Here's how the part is built. I have some questions about the finished solid (model axes, mm). A direction names the side the tool comes from. Coordinates: 2 decimals unless noted, no trailing zeros. Order: outer loops, then holes, each group sorted by start corner. A loop starts at its lowest first (then second) coordinate and runs counter-clockwise, first axis right, second up. Notation, with made-up numbers: (26.5, 80.5) - (56.5, 80.5) arc R18 cw to (56.5, 99.5) - close; hole circle Ø3 at (42, 66). An arc over 180 degrees is marked (long way). Answer in a Markdown table with one row per item. Add a question column.
Item 1: On a 3-axis mill with a long thin cutter (end or side, diameter ignored), from which of +Z, -Z, +X, -X, +Y, -Y can I reach the whole of each face in a straight line? I mean faces 1 (the flat face through (-2.4, -1, 0)), 2 (the flat face through (2.4, -1, 0)), 3 (the flat face through (-1, -2, 1)). Say none if no direction works.
Item 2: If I drill on line 1 along Z through (x, y) = (0, 0.5); line 2 along X through (y, z) = (-0.55, 0); line 3 along Y through (x, z) = (-5.5, 0.6), over which ranges is the centre line in solid material (lowest first)? Write a range as from..to.
Item 3: Thinking about a two-plate mould opening in Z: for faces 4 (the flat face through (0, 1, -3)), 5 (the cylindrical face through (-0.27, 0.28, 1.22)), 6 (the flat face through (0, 1, 3)), 7 (the flat face through (-6, 1, 0)), which applies, +Z half, -Z half, draft (parallel to the pull), parting line (faces both ways), or undercut?
Item 4: I want a section at D-D (z = -2.15). Please give me the cut outline in (x, y).
Item 5: I want a section at A-A (x = 0). Please give me the cut outline in (y, z), plus the area to 4 significant figures.
Item 6: Will these pins go through, and if not, where does the flat tip stop? pin 1 Ø1 at (y, z) = (-1, 1) entering from +X; pin 2 Ø1 at (x, z) = (4, -1) entering from -Y.
Item 7: I want a section at B-B (y = -1.7). Please give me the cut outline in (x, z), plus the area to 3 significant figures.
Item 8: I want a section at C-C (z = 0). Please give me the cut outline in (x, y), plus the area to 4 significant figures.
```python
from build123d import *

# Parameters (mm, degrees)
BOSS_EXTRU_1_DEPTH      = 3
ESQUISSE2_R             = 1.25
ENL_V_MAT_EXTRU_1_DEPTH = 5.5
CONG_1_R                = 0.5


with BuildPart() as part:
    # Esquisse1 → Boss.-Extru.1 (new body, symmetric)
    with BuildSketch(Plane.XY):
        Polygon((-6, 0), (-2.4, 0), (-2.4, -2), (2.4, -2), (2.4, 0), (6, 0), (6, 2.5), (-6, 2.5), align=None)
    extrude(amount=BOSS_EXTRU_1_DEPTH, both=True)

    # Esquisse2 → Enlèv. mat.-Extru.1 (cut, through all)
    with BuildSketch(Plane(origin=(0, 2.5, 0), x_dir=(1, 0, 0), z_dir=(0, 1, 0))):
        Circle(ESQUISSE2_R)
    extrude(amount=-ENL_V_MAT_EXTRU_1_DEPTH, mode=Mode.SUBTRACT)

    # Congé1
    cong_1_edges = [part.edges().sort_by_distance(p)[0] for p in [
        (-6, 1.25, -3),
        (6, 1.25, -3),
        (-6, 1.25, 3),
        (-2.4, -1, 3),
        (2.4, -1, 3),
        (6, 1.25, 3),
        (2.4, -1, -3),
        (-2.4, -1, -3),
    ]]
    fillet(cong_1_edges, radius=CONG_1_R)


solid = part.part
```
Values follow:
| question | item | result |
|---|---|---|
| 1 | face 1 | +Z, -Z, -X, -Y |
| 1 | face 2 | +Z, -Z, +X, -Y |
| 1 | face 3 | +Z, -Z, +X, -X, -Y |
| 2 | line 1 | z = -3..-1.25, 1.25..3 |
| 2 | line 2 | x = -2.4..-1.25, 1.25..2.4 |
| 2 | line 3 | y = 0..2.5 |
| 3 | face 4 | -Z half |
| 3 | face 5 | undercut |
| 3 | face 6 | +Z half |
| 3 | face 7 | draft |
| 4 | outline | (-6, 0) - (-2.4, 0) - (-2.4, -2) - (2.4, -2) - (2.4, 0) - (6, 0) - (6, 2.5) - (-6, 2.5) - close |
| 5 | outline | (-2, -3) - (2.5, -3) - (2.5, -1.25) - (-2, -1.25) - close; (-2, 1.25) - (2.5, 1.25) - (2.5, 3) - (-2, 3) - close |
| 5 | area | 15.75 mm^2 |
| 6 | pin 1 | stops at x = 2.4 |
| 6 | pin 2 | stops at y = 0 |
| 7 | outline | (-2.4, -2.5) arc R0.5 ccw to (-1.9, -3) - (1.9, -3) arc R0.5 ccw to (2.4, -2.5) - (2.4, 2.5) arc R0.5 ccw to (1.9, 3) - (-1.9, 3) arc R0.5 ccw to (-2.4, 2.5) - close; hole circle Ø2.5 at (0, 0) |
| 7 | area | 23.7 mm^2 |
| 8 | outline | (-6, 0) - (-2.4, 0) - (-2.4, -2) - (-1.25, -2) - (-1.25, 2.5) - (-6, 2.5) - close; (1.25, -2) - (2.4, -2) - (2.4, 0) - (6, 0) - (6, 2.5) - (1.25, 2.5) - close |
| 8 | area | 28.35 mm^2 |
